from build123d import *

# Parameters (mm, degrees)
SKETCH1_R           = 42.9384162
SKETCH1_R_2         = 39.624
BOSS_EXTRUDE1_DEPTH = 12.7
SKETCH4_R           = 1.692869147
CUT_EXTRUDE1_DEPTH  = 72.35
CIRPATTERN7_COUNT   = 3
SKETCH6_W           = 6.747965948
SKETCH6_H           = 12.700002404
BOSS_EXTRUDE2_DEPTH = 3.81
CIRPATTERN8_COUNT   = 4
CUT_EXTRUDE2_START  = -8.81
SKETCH7_R           = 1.692869147
CUT_EXTRUDE2_DEPTH  = 8.81
CUT_EXTRUDE3_START  = -24
CUT_EXTRUDE3_DEPTH  = 24


with BuildPart() as part:
    # Sketch1 → Boss-Extrude1 (new body)
    with BuildSketch(Plane(origin=(0, 0, 0), x_dir=(1, 0, 0), z_dir=(0, 1, 0))):
        with Locations(Location((0, 0, 0), (0, 0, 270))):
            Circle(SKETCH1_R)
        with Locations(Location((0, 0, 0), (0, 0, 270))):
            Circle(SKETCH1_R_2, mode=Mode.SUBTRACT)
    extrude(amount=BOSS_EXTRUDE1_DEPTH)

    # Sketch4 → Cut-Extrude1 (cut)
    with BuildSketch(Plane.XY):
        with Locations(Location((0, 3.287142885, 0), (0, 0, 180))):
            Circle(SKETCH4_R)
    cut_extrude1 = extrude(amount=CUT_EXTRUDE1_DEPTH, mode=Mode.SUBTRACT)

    # CirPattern7: Cut-Extrude1 ×3 about axis
    cirpattern7_axis = Axis((0, 0, 0), (0, -1, 0))
    for i in range(1, CIRPATTERN7_COUNT):
        add(cut_extrude1.rotate(cirpattern7_axis, i * 360 / CIRPATTERN7_COUNT), mode=Mode.SUBTRACT)

    # Sketch6 → Boss-Extrude2 (add, symmetric)
    with BuildSketch(Plane.XY):
        with Locations((45.914433226, 6.349998798)):
            Rectangle(SKETCH6_W, SKETCH6_H)
    boss_extrude2 = extrude(amount=BOSS_EXTRUDE2_DEPTH, both=True)

    # CirPattern8: Boss-Extrude2 ×4 about axis
    cirpattern8_axis = Axis((0, 0, 0), (0, 1, 0))
    for i in range(1, CIRPATTERN8_COUNT):
        add(boss_extrude2.rotate(cirpattern8_axis, i * 360 / CIRPATTERN8_COUNT))

    # Sketch7 → Cut-Extrude2 (cut)
    with BuildSketch(Plane.XY.offset(49.2884162).offset(CUT_EXTRUDE2_START)):
        with Locations(Location((0, 3.287142885, 0), (0, 0, 180))):
            Circle(SKETCH7_R)
    extrude(amount=CUT_EXTRUDE2_DEPTH, mode=Mode.SUBTRACT)

    # Sketch8 → Cut-Extrude3 (cut)
    with BuildSketch(Plane(origin=(0, 12.7, 0), x_dir=(1, 0, 0), z_dir=(0, 1, 0)).offset(CUT_EXTRUDE3_START)):
        with BuildLine():
            Line((-41.736458882, -3.81), (-42.769048222, -3.81))
            ThreePointArc((-42.769048222, -3.81), (-30.362045269, -30.362045269), (-3.81, -42.769048222))
            Line((-3.81, -42.769048222), (-3.81, -41.736458882))
            ThreePointArc((-3.81, -41.736458882), (-29.6348452, -29.6348452), (-41.736458882, -3.81))
        make_face()
        with BuildLine():
            Line((3.81, -41.736458882), (3.81, -42.769048222))
            ThreePointArc((3.81, -42.769048222), (30.362045269, -30.362045269), (42.769048222, -3.81))
            Line((42.769048222, -3.81), (41.736458882, -3.81))
            ThreePointArc((41.736458882, -3.81), (29.6348452, -29.6348452), (3.81, -41.736458882))
        make_face()
        with BuildLine():
            ThreePointArc((42.769048222, 3.81), (30.362045269, 30.362045269), (3.81, 42.769048222))
            Line((3.81, 42.769048222), (3.81, 41.736458882))
            ThreePointArc((3.81, 41.736458882), (29.6348452, 29.6348452), (41.736458882, 3.81))
            Line((41.736458882, 3.81), (42.769048222, 3.81))
        make_face()
        with BuildLine():
            ThreePointArc((-3.81, 42.769048222), (-30.362045269, 30.362045269), (-42.769048222, 3.81))
            Line((-42.769048222, 3.81), (-41.736458882, 3.81))
            ThreePointArc((-41.736458882, 3.81), (-29.6348452, 29.6348452), (-3.81, 41.736458882))
            Line((-3.81, 41.736458882), (-3.81, 42.769048222))
        make_face()
    extrude(amount=CUT_EXTRUDE3_DEPTH, mode=Mode.SUBTRACT)


solid = part.part
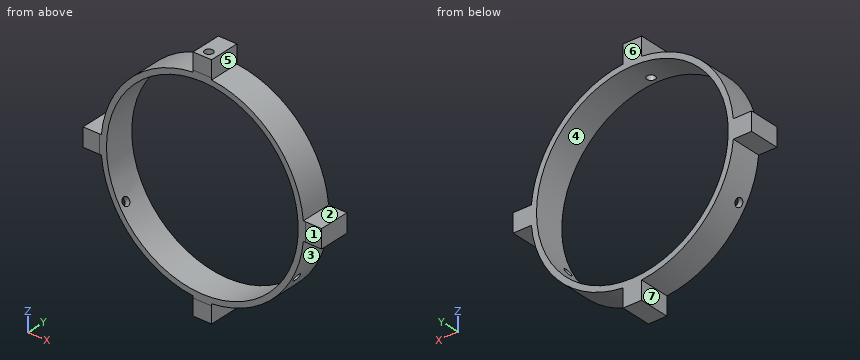
The listing builds one solid part. Answer for the finished solid, in the listing's coordinates (mm). Face numbers are marked on the shaded views. A direction names the side the tool comes from. Give positions to 0.01 mm unless a question says otherwise; leave off trailing zeros. Order: outer loops, then holes, each group sorted by start corner. A loop starts at its lowest first (then second) coordinate and runs counter-clockwise, first axis right, second up. Notation, with made-up numbers: (-10.5, 35.25) -> (26.5, 35.25) arc R27 ccw to (26.5, 65.25) -> close; hole circle Ø1 at (71, 17). An arc over 180 degrees is marked (long way). Put each result on its own line as item: value.
Item 1: Given P1, Ø4, axis at y = 9, z = -46.5, coming from the -X side; P2, Ø2.5, axis at y = 4, z = 44, coming from the +X side; P3, Ø4, axis at x = 44.5, y = 5, coming from the -Z side, each flat-ended and moving along its own axis, determine where each tip first touches the part or whether it passes through.
Established:
P1: stops at x = -3.81
P2: stops at x = 3.81
P3: stops at z = -3.81
Item 2: A cutting plane is placed at D-D on z = 17.5. Give the vertices of the cut face in (x, y).
Established:
outline: (-38.08, 0) -> (-35.55, 0) -> (-35.55, 12.7) -> (-38.08, 12.7) -> close; (35.55, 0) -> (38.08, 0) -> (38.08, 12.7) -> (35.55, 12.7) -> close
Item 3: Straight lines are drawn through the part: line 1 (Y direction, x = 0, z = 44); line 2 (X direction, y = 8.75, z = 0); line 3 (X direction, y = 1.5, z = 43.5). For each, find the intervals that lie inside material, in ascending order.
Established:
line 1: y = 0 to 1.59, 4.98 to 12.7
line 2: x = -49.29 to -39.62, 39.62 to 49.29
line 3: x = -3.81 to 3.81
Item 4: For the marked faces 5, 6 and 7, determine the directions among +Z, -Z, +X, -X, +Y, -Y from which every point of the face is accessible in a straight line to the end or side of a thin tool.
Established:
face 5: +Z, +X, +Y, -Y
face 6: +Z, -Z, +X, -X, +Y
face 7: -Z, -X, +Y, -Y
Item 5: A cutting plane is placed at C-C on x = -31.5. Give the vertices of the cut face in (y, z), plus the area to 3 significant figures.
Established:
outline: (0, -27.64) -> (12.7, -27.64) -> (12.7, -24.04) -> (0, -24.04) -> close; (0, 24.04) -> (12.7, 24.04) -> (12.7, 27.64) -> (0, 27.64) -> close
area: 91.6 mm^2
Item 6: For a pull along Z with two mould halves and no side action, classify the marked faces 1, 2, 3 and 4 as released by +Z, released by -Z, zero draft, split by the parting line, or undercut.
Established:
face 1: zero draft
face 2: released by +Z
face 3: released by -Z
face 4: undercut
Item 7: A cutting plane is placed at B-B on x = 0. Count the separate pieces of the cut face and the enclosed holes in it, plus the area to 3 significant figures.
Established:
separate pieces: 3
enclosed holes: 0
area: 213 mm^2
